from build123d import *

# Parameters (mm, degrees)
SKETCH_1_R      = 2
EXTRUDE_1_DEPTH = 5


with BuildPart() as part:
    # 草图1 → 凸台-拉伸1 (new body)
    with BuildSketch(Plane(origin=(0, 0, 0), x_dir=(1, 0, 0), z_dir=(0, 1, 0))):
        with BuildLine():
            ThreePointArc((-53.6685, 4), (-54.272481718, 3.954137843), (-54.862613484, 3.817603042))
            ThreePointArc((-54.862613484, 3.817603042), (-57.622637843, -0.603981718), (-53.6685, -4))
            ThreePointArc((-53.6685, -4), (-53.064518282, -3.954137843), (-52.474386516, -3.817603042))
            Line((-52.474386516, -3.817603042), (-27.481364025, 4))
            Line((-27.481364025, 4), (-53.6685, 4))
        make_face()
        with Locations((-53.6685, 0)):
            Circle(SKETCH_1_R, mode=Mode.SUBTRACT)
        with BuildLine():
            Line((4.544386516, 22.399603042), (-54.862613484, 3.817603042))
            ThreePointArc((-54.862613484, 3.817603042), (-54.272481718, 3.954137843), (-53.6685, 4))
            Line((-53.6685, 4), (-27.481364025, 4))
            Line((-27.481364025, 4), (5.597201207, 14.346691453))
            Line((5.597201207, 14.346691453), (4.292598412, 14.852473408))
            ThreePointArc((4.292598412, 14.852473408), (1.740724203, 18.715374202), (4.544386516, 22.399603042))
        make_face()
        with BuildLine():
            ThreePointArc((7.184401588, 22.311526592), (5.871874202, 22.579775797), (4.544386516, 22.399603042))
            ThreePointArc((4.544386516, 22.399603042), (1.740724203, 18.715374202), (4.292598412, 14.852473408))
            Line((4.292598412, 14.852473408), (5.597201207, 14.346691453))
            Line((5.597201207, 14.346691453), (6.932613484, 14.764396958))
            ThreePointArc((6.932613484, 14.764396958), (9.736275797, 18.448625798), (7.184401588, 22.311526592))
        make_face()
        with Locations((5.7385, 18.582)):
            Circle(SKETCH_1_R, mode=Mode.SUBTRACT)
        with BuildLine():
            Line((55.114401588, 3.729526592), (7.184401588, 22.311526592))
            ThreePointArc((7.184401588, 22.311526592), (9.736275797, 18.448625798), (6.932613484, 14.764396958))
            Line((6.932613484, 14.764396958), (5.597201207, 14.346691453))
            Line((5.597201207, 14.346691453), (32.285228401, 4))
            Line((32.285228401, 4), (53.6685, 4))
            ThreePointArc((53.6685, 4), (54.403990868, 3.931800247), (55.114401588, 3.729526592))
        make_face()
        with BuildLine():
            ThreePointArc((-52.474386516, -3.817603042), (-53.064518282, -3.954137843), (-53.6685, -4))
            Line((-53.6685, -4), (53.6685, -4))
            ThreePointArc((53.6685, -4), (52.933009132, -3.931800247), (52.222598412, -3.729526592))
            Line((52.222598412, -3.729526592), (32.285228401, 4))
            Line((32.285228401, 4), (-27.481364025, 4))
            Line((-27.481364025, 4), (-52.474386516, -3.817603042))
        make_face()
        with BuildLine():
            ThreePointArc((52.222598412, -3.729526592), (52.933009132, -3.931800247), (53.6685, -4))
            ThreePointArc((53.6685, -4), (57.600300247, -0.735490868), (55.114401588, 3.729526592))
            ThreePointArc((55.114401588, 3.729526592), (54.403990868, 3.931800247), (53.6685, 4))
            Line((53.6685, 4), (32.285228401, 4))
            Line((32.285228401, 4), (52.222598412, -3.729526592))
        make_face()
        with Locations((53.6685, 0)):
            Circle(SKETCH_1_R, mode=Mode.SUBTRACT)
        Polygon((5.597201207, 14.346691453), (-27.481364025, 4), (32.285228401, 4), align=None)
        with Locations((-53.6685, 0)):
            Circle(SKETCH_1_R)
    extrude(amount=EXTRUDE_1_DEPTH)


solid = part.part
Here's how the part is built. I have some questions about the finished solid (model axes, mm). Round coordinates to 2 decimals unless told otherwise and drop trailing zeros. Loops run counter-clockwise (first coordinate to the right, second up) from the corner with the lowest first, then second, coordinate; pieces in that order, holes last.
1. If we section it at A-A on z = 0: Write out the boundary of the cut face in (x, y).
Answer list:
outline: (-57.67, 0) - (51.67, 0) - (51.67, 5) - (-57.67, 5) - close; (55.67, 0) - (57.67, 0) - (57.67, 5) - (55.67, 5) - close
2. If I drill on line 1 along X through (y, z) = (2.8, 0); line 2 along Z through (x, y) = (-33.5, 0.8); line 3 along Z through (x, y) = (-6.5, 3.95), over which ranges is the centre line in solid material (lowest first)?
Answer list:
line 1: x = -57.67 to 51.67, 55.67 to 57.67
line 2: z = -10.5 to 4
line 3: z = -18.95 to 4
3. If we section it at B-B on y = 2: Write out the boundary of the cut face in (x, z).
Answer list:
outline: (-54.86, -3.82) - (4.54, -22.4) arc R4 ccw to (7.18, -22.31) - (55.11, -3.73) arc R4 ccw to (53.67, 4) - (-53.67, 4) arc R4 ccw to start; hole circle Ø4 at (5.74, -18.58); hole circle Ø4 at (53.67, 0)
4. If we section it at C-C on x = 36.5: Write out the boundary of the cut face in (y, z).
Answer list:
outline: (0, -10.95) - (5, -10.95) - (5, 4) - (0, 4) - close
5. For P1, Ø3.5, axis at x = 5.74, z = -18.58, coming from the +Y side; P2, Ø1.5, axis at x = -43, y = 0.5, coming from the -Z side; P3, Ø3, axis at x = 12.5, y = 4, coming from the -Z side; P4, Ø2, axis at x = -8.5, y = 2, coming from the -Z side, each with a flat end and sliding along its axis, tell me the tip position at first contact or that it passes through.
Answer list:
P1: passes through
P2: stops at z = -7.76
P3: stops at z = -20.83
P4: stops at z = -18.63
6. We'd pull the mould along Z, two halves only. Please class faces 1 (the face through (5.89, 2.46, -22.58)), 2 (the face through (6.661, 2.465, -16.808)), 3 (the face through (-1, 0, -7)): +Z half, -Z half, draft (parallel to the pull), parting line (faces both ways), or undercut.
Answer list:
face 1: -Z half
face 2: undercut
face 3: draft
7. If we section it at D-D on z = -8.25: Write out the boundary of the cut face in (x, y), plus the area to 3 significant figures.
Answer list:
outline: (-40.69, 0) - (43.45, 0) - (43.45, 5) - (-40.69, 5) - close
area: 421 mm2
